Geometry: see drawing. Coordinates: mm, zero at the bounding-box minimum. A direction names the side the tool comes from. Coordinates: 2 decimals unless noted, no trailing zeros. Order: outer loops, then holes, each group sorted by start corner. A loop starts at its lowest first (then second) coordinate and runs counter-clockwise, first axis right, second up.
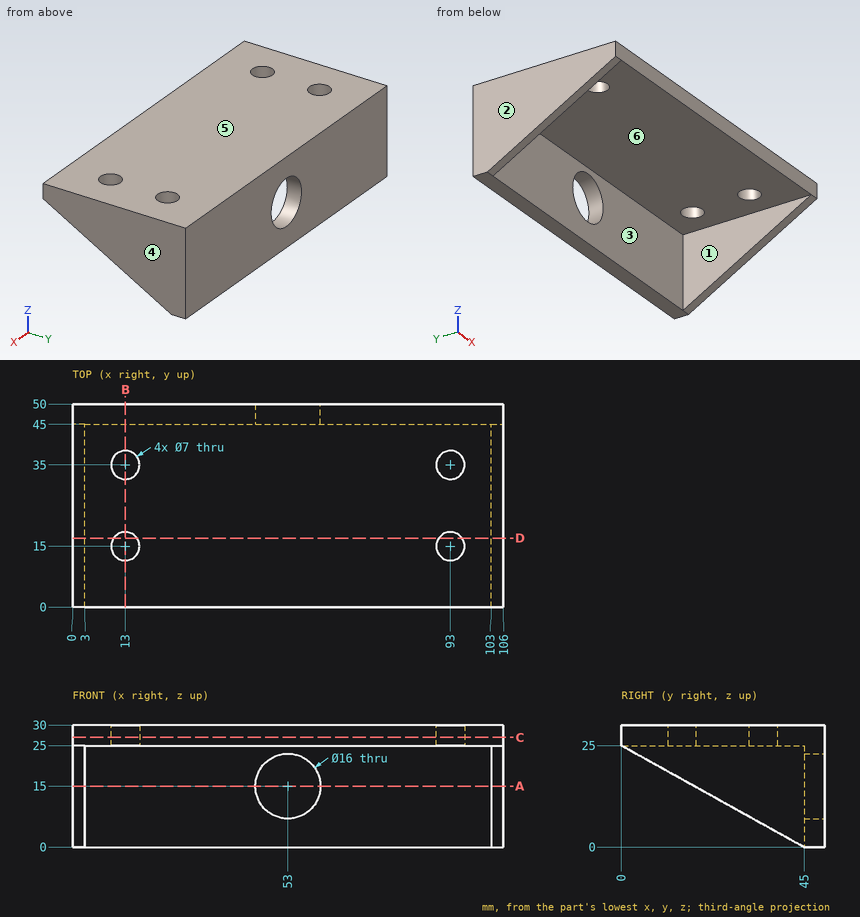
Item 1: Cut plane C-C on z = 27. Return loops of the section in (x, y), then the cut area to 3 significant figures.
Response values:
outline: (0, 0) - (106, 0) - (106, 50) - (0, 50) - close; hole circle Ø7 at (13, 15); hole circle Ø7 at (13, 35); hole circle Ø7 at (93, 15); hole circle Ø7 at (93, 35)
area: 5,150 mm2
Item 2: Cut plane D-D on y = 17. Return loops of the section in (x, z).
Response values:
outline: (0, 15.56) - (3, 15.56) - (3, 25) - (10.13, 25) - (10.13, 30) - (0, 30) - close; (15.87, 25) - (90.13, 25) - (90.13, 30) - (15.87, 30) - close; (95.87, 25) - (103, 25) - (103, 15.56) - (106, 15.56) - (106, 30) - (95.87, 30) - close
Item 3: Draft query along X for the marked faces 1, 2, 3 and 4. Return one class per face: pulls with the +X half, pulls with the -X half, needs draft (parallel to the pull), parting line crosses it, or undercut.
Response values:
face 1: undercut
face 2: pulls with the -X half
face 3: undercut
face 4: pulls with the +X half
Item 4: Ray query, probe 1 along Y at (x, z) = (93, 26); probe 2 along X at (y, z) = (44.5, 8); probe 3 along Z at (x, y) = (53, 47.8). Return the intervals inside material, ascending.
Response values:
probe 1: y = 0 to 11.5, 18.5 to 31.5, 38.5 to 50
probe 2: x = 0 to 3, 103 to 106
probe 3: z = 0 to 7, 23 to 30
Item 5: Pin query (flat end, axial travel): pin 1 Ø1.5 at (x, y) = (40.5, 39) entering from -Z; pin 2 Ø1.5 at (x, z) = (24, 5.5) entering from -Y; pin 3 Ø4 at (x, y) = (93, 35) entering from -Z; pin 4 Ø1 at (x, z) = (47.5, 9.5) entering from +Y. Return the tip coordinate at first contact, or that it passes through.
Response values:
pin 1: stops at z = 25
pin 2: stops at y = 45
pin 3: passes through
pin 4: stops at y = 50
Item 6: Access query for the marked faces 5 and 6. Directions: +Z, -Z, +X, -X, +Y, -Y. A direction counts if a zero-diameter tool reaches every point of the face in a straight line with its end or side. Return the directions, or none.
Response values:
face 5: +Z, +X, -X, +Y, -Y
face 6: -Z, -Y
Item 7: Cut plane A-A on z = 15. Return loops of the section in (x, y), then the cut area to 3 significant figures.
Response values:
outline: (0, 18) - (3, 18) - (3, 45) - (45, 45) - (45, 50) - (0, 50) - close; (61, 45) - (103, 45) - (103, 18) - (106, 18) - (106, 50) - (61, 50) - close
area: 612 mm2
Item 8: Cut plane B-B on x = 13. Return loops of the section in (y, z).
Response values:
outline: (0, 25) - (11.5, 25) - (11.5, 30) - (0, 30) - close; (18.5, 25) - (31.5, 25) - (31.5, 30) - (18.5, 30) - close; (38.5, 25) - (45, 25) - (45, 0) - (50, 0) - (50, 30) - (38.5, 30) - close
